Can you work these out from the model? Positions are in its coordinate system, mm. A direction names the side the tool comes from. Round coordinates to 2 decimals unless told otherwise and drop trailing zeros. Order: outer loops, then holes, each group sorted by start corner. A loop starts at its lowest first (then second) coordinate and runs counter-clockwise, first axis right, second up. Notation, with made-up numbers: M 39,3 L 58,3 A30 ccw 58,40 Z; hole C 54.25,11.5 d10. An arc over 180 degrees is marked long. One line per question, with ' | ' between items.
```python
from build123d import *

# Parameters (mm, degrees)
EXTRUDE_1_DEPTH          = 25
CUT_EXTRUDE_1_DEPTH      = 100
CUT_EXTRUDE_1_DEPTH_BACK = 100
SKETCH_2_W               = 3
SKETCH_2_H               = 15
SKETCH_5_W               = 60
SKETCH_5_H               = 45
EXTRUDE_2_DEPTH          = 15
SKETCH_7_W               = 2
SKETCH_7_H               = 11
CUT_EXTRUDE_2_DEPTH      = 103
CUT_EXTRUDE_3_DEPTH      = 103
CUT_EXTRUDE_4_DEPTH      = 103
EXTRUDE_4_DEPTH          = 62
CUT_EXTRUDE_5_DEPTH      = 30
CUT_EXTRUDE_5_DEPTH_BACK = 123
SKETCH_15_R              = 6
CUT_EXTRUDE_6_DEPTH      = 4
SKETCH_18_W              = 40
SKETCH_18_H              = 14.629062191
EXTRUDE_5_DEPTH          = 5
SKETCH_19_R              = 40
SKETCH_19_R_2            = 5
EXTRUDE_7_DEPTH          = 10
SKETCH_19_8_R            = 15
CUT_EXTRUDE_8_DEPTH      = 25


with BuildPart() as part:
    # Sketch 1 → Extrude 1 (new body)
    with BuildSketch(Plane.XY):
        Polygon((20, 0), (25, 0), (25, 50), (0, 50), (0, 45), (20, 45), align=None)
        Polygon((-25, 50), (-25, 0), (-20, 0), (-20, 45), (0, 45), (0, 50), align=None)
        Polygon((-25, -50), (0, -50), (0, -45), (-20, -45), (-20, 0), (-25, 0), align=None)
        Polygon((0, -45), (0, -50), (25, -50), (25, 0), (20, 0), (20, -45), align=None)
    extrude(amount=EXTRUDE_1_DEPTH)

    # Sketch 2 → Cut-Extrude 1 (cut, two sides: drawn at the far end of the back side and taken through both)
    with BuildSketch(Plane(origin=(0, 0, 0), x_dir=(1, 0, 0), z_dir=(0, 1, 0)).offset(-CUT_EXTRUDE_1_DEPTH_BACK)):
        with Locations((23.5, -17.5)):
            Rectangle(SKETCH_2_W, SKETCH_2_H)
        with Locations((-23.5, -17.5)):
            Rectangle(SKETCH_2_W, SKETCH_2_H)
    extrude(amount=CUT_EXTRUDE_1_DEPTH + CUT_EXTRUDE_1_DEPTH_BACK, mode=Mode.SUBTRACT)

    # Sketch 5 → Extrude 2 (add)
    with BuildSketch(Plane(origin=(0, 50, 0), x_dir=(1, 0, 0), z_dir=(0, 1, 0))):
        with Locations((0, -4.5)):
            Rectangle(SKETCH_5_W, SKETCH_5_H)
    extrude(amount=EXTRUDE_2_DEPTH)

    # Sketch 7 → Cut-Extrude 2 (cut)
    with BuildSketch(Plane.ZY.offset(30)):
        with Locations((26, 59.5)):
            Rectangle(SKETCH_7_W, SKETCH_7_H)
    extrude(amount=-CUT_EXTRUDE_2_DEPTH, mode=Mode.SUBTRACT)

    # Sketch 12 → Cut-Extrude 3 (cut)
    with BuildSketch(Plane.ZY.offset(30)):
        Polygon((-9.968923852, 65), (-18, 54), (-18, 65), align=None)
    extrude(amount=-CUT_EXTRUDE_3_DEPTH, mode=Mode.SUBTRACT)

    # Sketch 13 → Cut-Extrude 4 (cut)
    with BuildSketch(Plane.ZY.offset(30)):
        Polygon((0, 50), (0, 54), (-18, 54), (-18, 49.192005068), (0, 49.192005068), align=None)
    extrude(amount=-CUT_EXTRUDE_4_DEPTH, mode=Mode.SUBTRACT)

    # Sketch 14 → Extrude 4 (add)
    with BuildSketch(Plane.ZY.offset(31)):
        with BuildLine():
            Line((-1, 49), (0, 49))
            Line((0, 49), (0, 53))
            ThreePointArc((0, 53), (-0.292893219, 53.707106781), (-1, 54))
            Line((-1, 54), (-19, 54))
            Line((-19, 54), (-19, 53))
            Line((-19, 53), (-1, 53))
            Line((-1, 53), (-1, 49))
        make_face()
    extrude(amount=-EXTRUDE_4_DEPTH)

    # Sketch 15 → Cut-Extrude 5 (cut, two sides: drawn at the far end of the back side and taken through both)
    with BuildSketch(Plane(origin=(0, 50, 0), x_dir=(1, 0, 0), z_dir=(0, 1, 0)).offset(-CUT_EXTRUDE_5_DEPTH_BACK)):
        with Locations(Location((0, -10, 0), (0, 0, 270))):
            Circle(SKETCH_15_R)
    extrude(amount=CUT_EXTRUDE_5_DEPTH + CUT_EXTRUDE_5_DEPTH_BACK, mode=Mode.SUBTRACT)

    # Sketch 16 → Cut-Extrude 6 (cut)
    with BuildSketch(Plane.XZ.offset(-53)):
        with BuildLine():
            Line((12, -10), (15, -10))
            Line((15, -10), (18, -10))
            ThreePointArc((18, -10), (15, -7), (12, -10))
        make_face()
        with BuildLine():
            Line((18, -10), (15, -10))
            Line((15, -10), (12, -10))
            ThreePointArc((12, -10), (15, -13), (18, -10))
        make_face()
        with BuildLine():
            ThreePointArc((-18, -10), (-15, -13), (-12, -10))
            Line((-12, -10), (-15, -10))
            Line((-15, -10), (-18, -10))
        make_face()
        with BuildLine():
            Line((-15, -10), (-12, -10))
            ThreePointArc((-12, -10), (-15, -7), (-18, -10))
            Line((-18, -10), (-15, -10))
        make_face()
    extrude(amount=-CUT_EXTRUDE_6_DEPTH, mode=Mode.SUBTRACT)

    # Sketch 18 → Extrude 5 (add)
    with BuildSketch(Plane.XY.offset(25)):
        with Locations((0, 37.685468904)):
            Rectangle(SKETCH_18_W, SKETCH_18_H)
    extrude(amount=-EXTRUDE_5_DEPTH)

    # Sketch 19 → Extrude 7 (add)
    with BuildSketch(Plane.XY.offset(25)):
        with Locations(Location((0, 5.916189744, 0), (0, 0, 236.632987031))):
            Circle(SKETCH_19_R)
        with Locations((0, 35.916189744)):
            Circle(SKETCH_19_R_2, mode=Mode.SUBTRACT)
        with Locations((30, 5.916189744)):
            Circle(SKETCH_19_R_2, mode=Mode.SUBTRACT)
        with Locations((0, -24.083810256)):
            Circle(SKETCH_19_R_2, mode=Mode.SUBTRACT)
        with Locations((-30, 5.916189744)):
            Circle(SKETCH_19_R_2, mode=Mode.SUBTRACT)
    extrude(amount=EXTRUDE_7_DEPTH)

    # Sketch 19_8 → Cut-Extrude 8 (cut)
    with BuildSketch(Plane.XY.offset(25)):
        with Locations(Location((0, 5.916189744, 0), (0, 0, 180))):
            Circle(SKETCH_19_8_R)
    extrude(amount=CUT_EXTRUDE_8_DEPTH, mode=Mode.SUBTRACT)


solid = part.part
```
(1) Will these pins go through, and if not, where does the flat tip stop? pin 1 Ø20 at (x, y) = (4.5, 6) entering from -Z; pin 2 Ø2.5 at (y, z) = (52, -6) entering from -X; pin 3 Ø7.5 at (y, z) = (58.5, -3.5) entering from +X; pin 4 Ø2 at (x, y) = (27.5, 51.5) entering from +Z.
Final values:
pin 1: through | pin 2: x = -31 | pin 3: x = 30 | pin 4: z = 27
(2) Thinking about a two-plate mould opening in Y: for faces 5 (the flat face through (0, 53, -10)), 6 (the flat face through (-14, 16, 35)), 7 (the flat face through (-0.1, 50, 25.4)), 8 (the cylindrical face through (-0.651, -19.126, 29.93)), which applies, released by +Y, released by -Y, zero draft, split by the parting line, or undercut?
Final values:
face 5: released by -Y | face 6: zero draft | face 7: undercut | face 8: undercut
(3) On a 3-axis mill with a long thin cutter (end or side, diameter ignored), from which of +Z, -Z, +X, -X, +Y, -Y can I reach the whole of each face in a straight line? I mean faces 1 (the flat face through (20.3, -4.4, 0)), 2 (the flat face through (-24, -1, 10)), 3 (the flat face through (30, 57, 10)), 4 (the flat face through (-30, 57, 10)). Say none if no direction works.
Final values:
face 1: -Z, +X, -X, -Y | face 2: -X, -Y | face 3: +Z, +X, +Y | face 4: +Z, -X, +Y
(4) If we section it at D-D on y = 33.5: Please give me the cut outline in (x, z).
Final values:
outline: M -28.97,25 L -22,25 L -22,10 L -25,10 L -25,0 L -20,0 L -20,20 L 20,20 L 20,0 L 25,0 L 25,10 L 22,10 L 22,25 L 28.97,25 L 28.97,35 L 4.38,35 L 4.38,25 L -4.38,25 L -4.38,35 L -28.97,35 Z
(5) If we section it at C-C on z = 12: Please give me the cut outline in (x, y).
Final values:
outline: M -30,50 L -22,50 L -22,-50 L -5.66,-50 L -5.66,-45 L -20,-45 L -20,45 L -5.66,45 L -5.66,65 L -30,65 Z; M 5.66,-50 L 22,-50 L 22,50 L 30,50 L 30,65 L 5.66,65 L 5.66,45 L 20,45 L 20,-45 L 5.66,-45 Z
(6) If we section it at B-B on y = -3.5: Please give me the cut outline in (x, z).
Final values:
outline: M -38.88,25 L -22,25 L -22,10 L -25,10 L -25,0 L -20,0 L -20,25 L -11.68,25 L -11.68,35 L -38.88,35 Z; M 11.68,25 L 20,25 L 20,0 L 25,0 L 25,10 L 22,10 L 22,25 L 38.88,25 L 38.88,35 L 11.68,35 Z
(7) Please list where these lines run through material, in increasing order: probe 1 along Y at (x, z) = (0, 29); probe 2 along Z at (x, y) = (24.5, -1.5); probe 3 along X at (y, z) = (-44, 17.5). Write a range as [from, to].
Final values:
probe 1: [-34.08, -29.08], [-19.08, -9.08], [20.92, 30.92], [40.92, 45.92] | probe 2: [0, 10], [25, 35] | probe 3: [-22, -20], [20, 22]
(8) If we section it at A-A on x = 0: State how many separate pieces and enclosed holes the cut face has, plus the area to 3 significant figures.
Final values:
separate pieces: 6 | enclosed holes: 1 | area: 883 mm^2
